For this review, take the finished solid that the model builds, in its own axes (mm). Give positions to 0.01 mm unless a question says otherwise; leave off trailing zeros. Loops run counter-clockwise (first coordinate to the right, second up) from the corner with the lowest first, then second, coordinate; pieces in that order, holes last. Notation, with made-up numbers: (85, 3) - (141, 3) arc R8 ccw to (141, 14) - close; hole circle Ø9 at (77.5, 78.25). An arc over 180 degrees is marked (long way). Use CSV: the item, a comma, the result in double quotes. Start each with the question number.
1. Wall thickness on line 1 (X direction, y = 0, z = 0.9); line 2 (Y direction, x = 14, z = 0.15); line 3 (Y direction, x = -0.5, z = 1.95): over which ranges is each line inside the solid? List them lowest first.
2. For pin 1 (3 mm diameter, centred on x = 14, y = 0, fed in from -Z), flat-tipped, find the tip position at first contact; note if it passes through.
3. Take a section at B-B on y = 0. State how many separate pieces and enclosed holes the cut face has, plus the area to 3 significant figures.
4. Take a section at A-A on z = 0.65. Give the boundary of the cut face in (x, y), plus the area to 3 significant figures.
5. Take a section at D-D on y = 24. Give the boundary of the cut face in (x, z).
```python
from build123d import *

# Parameters (mm, degrees)
SKETCH_W        = 36
SKETCH_H        = 56
PAD_DEPTH       = 2
SKETCH001_R     = 2
POCKET_DEPTH    = 3
CHAMFER_SIZE    = 1.99
POCKET001_DEPTH = 3


with BuildPart() as part:
    # Sketch → Pad (new body)
    with BuildSketch(Plane.XY):
        Rectangle(SKETCH_W, SKETCH_H)
    extrude(amount=PAD_DEPTH)

    # Sketch001 (on Face5 of Pad) → Pocket (cut)
    with BuildSketch(Plane(origin=(0, 0, 0), x_dir=(1, 0, 0), z_dir=(0, 0, -1))):
        with Locations((14, 0)):
            Circle(SKETCH001_R)
        with Locations((-14, 0)):
            Circle(SKETCH001_R)
    extrude(amount=-POCKET_DEPTH, mode=Mode.SUBTRACT)

    # Chamfer
    chamfer_edges = [part.edges().sort_by_distance(p)[0] for p in [
        (-16, 0, 0),
        (12, 0, 0),
    ]]
    chamfer(chamfer_edges, length=CHAMFER_SIZE)

    # Sketch002 (on Face1 of Chamfer) → Pocket001 (cut)
    with BuildSketch(Plane(origin=(0, 0, 0), x_dir=(1, 0, 0), z_dir=(0, 0, -1))):
        with BuildLine():
            ThreePointArc((2.49784, -22.5), (0, -20.103904), (-2.49784, -22.5))
            Line((-2.49784, -22.5), (-2.5, -28))
            Line((-2.5, -28), (2.5, -28))
            Line((2.49784, -22.5), (2.5, -28))
        make_face()
    extrude(amount=-POCKET001_DEPTH, mode=Mode.SUBTRACT)


solid = part.part
```
Check result:
1,line 1,"x = -18 to -17.09, -10.91 to 10.91, 17.09 to 18"
1,line 2,"y = -28 to -3.84, 3.84 to 28"
1,line 3,"y = -28 to 20.15"
2,pin 1,"passes through"
3,separate pieces,"3"
3,enclosed holes,"0"
3,area,"48.1 mm²"
4,outline,"(-18, -28) - (18, -28) - (18, 28) - (2.5, 28) - (2.5, 22.5) arc R2.5 cw to (-2.5, 22.5) - (-2.5, 28) - (-18, 28) - close; hole circle Ø6.68 at (-14, 0); hole circle Ø6.68 at (14, 0)"
4,area,"1,910 mm²"
5,outline,"(-18, 0) - (-2.5, 0) - (-2.5, 2) - (-18, 2) - close; (2.5, 0) - (18, 0) - (18, 2) - (2.5, 2) - close"
